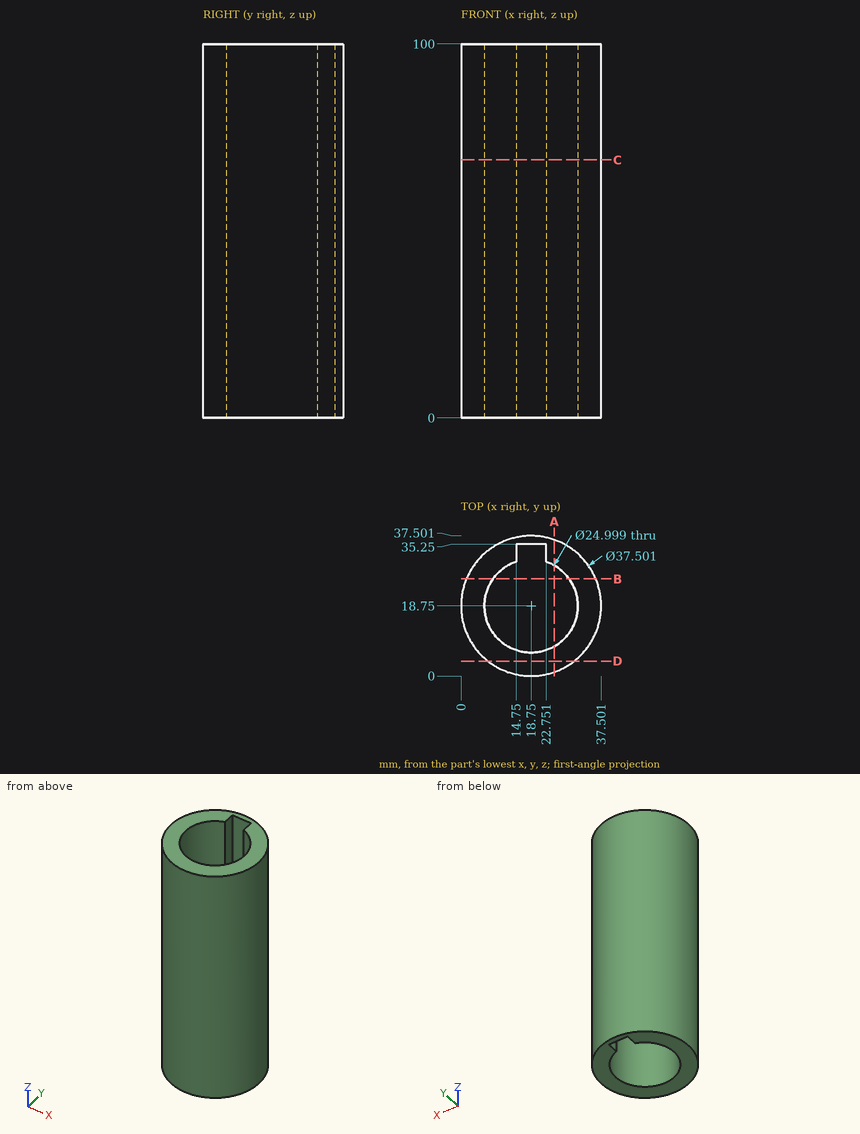
Input: dimensioned drawing with shaded views. Units: mm. Origin: part minimum x, y, z. Coordinates: 2 decimals unless noted, no trailing zeros. Loops run counter-clockwise (first coordinate to the right, second up) from the corner with the lowest first, then second, coordinate; pieces in that order, holes last. Notation, with made-up numbers: (30.25, 40.25) -> (69.25, 40.25) arc R26 ccw to (69.25, 63.25) -> close; hole circle Ø3 at (-2, -1). An arc over 180 degrees is marked (long way). Use a Markdown table: item, result. Add a question column.
(1) Section query D-D, the plane y = 4. Return loops of the section in (x, z) (1 decimal).
(2) Line query: line 1 along X through (y, z) = (9, 92) (1 decimal); line 2 along Y through (x, z) = (29.5, 48.5) (1 decimal); line 3 along X through (y, z) = (16.5, 8.5) (1 decimal). Output: solid intervals per line, ascending.
(3) Pin query (flat end, axial travel): pin 1 Ø3.5 at (y, z) = (32, 41.5) entering from +X; pin 2 Ø1 at (x, z) = (33, 81) entering from -Y; pin 3 Ø2.5 at (y, z) = (32.5, 31) entering from -X (1 decimal). Return the tip coordinate at first contact, or that it passes through.
(4) Section query A-A, the plane x = 25. Return loops of the section in (y, z) (1 decimal), plus the area to 3 significant figures.
(5) Section query B-B, the plane y = 26. Return loops of the section in (x, z), plus the area to 3 significant figures.
(6) Section query C-C, the plane z = 69. Return loops of the section in (x, y).
Answer:
| question | item | result |
|---|---|---|
| 1 | outline | (7.2, 0) -> (30.3, 0) -> (30.3, 100) -> (7.2, 100) -> close |
| 2 | line 1 | x = 2.7 to 10.9, 26.6 to 34.8 |
| 2 | line 2 | y = 3.4 to 12.4, 25.1 to 34.1 |
| 2 | line 3 | x = 0.1 to 6.5, 31 to 37.4 |
| 3 | pin 1 | stops at x = 33.56 |
| 3 | pin 2 | stops at y = 6 |
| 3 | pin 3 | stops at x = 4.8 |
| 4 | outline | (1.1, 0) -> (7.9, 0) -> (7.9, 100) -> (1.1, 100) -> close; (29.6, 0) -> (36.4, 0) -> (36.4, 100) -> (29.6, 100) -> close |
| 4 | area | 1,370 mm^2 |
| 5 | outline | (1.46, 0) -> (8.57, 0) -> (8.57, 100) -> (1.46, 100) -> close; (28.93, 0) -> (36.04, 0) -> (36.04, 100) -> (28.93, 100) -> close |
| 5 | area | 1,420 mm^2 |
| 6 | outline | circle Ø37.5 at (18.75, 18.75); hole (14.75, 30.59) arc R12.5 ccw (long way) to (22.75, 30.59) -> (22.75, 35.25) -> (14.75, 35.25) -> close |
